```python
from build123d import *

# Parameters (mm, degrees)
ESTRUSIONE_ESTRUSIONE1_DEPTH = 60
SCHIZZO2_R                   = 2.6
TAGLIO_ESTRUSIONE1_DEPTH     = 60
SCHIZZO3_R                   = 2.4
TAGLIO_ESTRUSIONE2_DEPTH     = 10


with BuildPart() as part:
    # Schizzo1 → Estrusione-Estrusione1 (new body)
    with BuildSketch(Plane.XY):
        with BuildLine():
            Line((7.046874237, -2.567404038), (4.547114317, -1.124166975))
            Line((4.547114317, -1.124166975), (3.247114317, -3.375833025))
            Line((3.247114317, -3.375833025), (5.746874237, -4.819070087))
            ThreePointArc((5.746874237, -4.819070087), (0, -7.5), (-5.746874237, -4.819070087))
            Line((-5.746874237, -4.819070087), (-3.247114317, -3.375833025))
            Line((-3.247114317, -3.375833025), (-4.547114317, -1.124166975))
            Line((-4.547114317, -1.124166975), (-7.046874237, -2.567404038))
            ThreePointArc((-7.046874237, -2.567404038), (-6.495190528, 3.75), (-1.3, 7.386474125))
            Line((-1.3, 7.386474125), (-1.3, 4.5))
            Line((-1.3, 4.5), (1.3, 4.5))
            Line((1.3, 4.5), (1.3, 7.386474125))
            ThreePointArc((1.3, 7.386474125), (6.495190528, 3.75), (7.046874237, -2.567404038))
        make_face()
    extrude(amount=ESTRUSIONE_ESTRUSIONE1_DEPTH)

    # Schizzo2 → Taglio-Estrusione1 (cut)
    with BuildSketch(Plane.XY.offset(60)):
        Circle(SCHIZZO2_R)
    extrude(amount=-TAGLIO_ESTRUSIONE1_DEPTH, mode=Mode.SUBTRACT)

    # Schizzo3 → Taglio-Estrusione2 (cut)
    with BuildSketch(Plane(origin=(0, 0, 0), x_dir=(1, 0, 0), z_dir=(0, 1, 0))):
        with Locations(Location((0, -30, 0), (0, 0, 270))):
            Circle(SCHIZZO3_R)
    extrude(amount=-TAGLIO_ESTRUSIONE2_DEPTH, mode=Mode.SUBTRACT)


solid = part.part
```
Read the model definition and answer for the solid it produces. Units are mm, in the model's axes. A direction names the side the tool comes from. Round coordinates to 2 decimals unless told otherwise and drop trailing zeros. Write each loop counter-clockwise with the first axis right and the second up, starting at its lowest first coordinate (ties: lowest second). Pieces come first, ordered by that corner, then holes. Notation, with made-up numbers: (22.5, -16) - (80.5, -16) arc R18 ccw to (80.5, 5) - close; hole circle Ø3 at (-36, 0.25). An arc over 180 degrees is marked (long way). Use CSV: the item, a comma, the result in double quotes.
Q1. Each of these flat-tipped pins is pushed along its axis until it touches: pin 1 Ø1 at (x, z) = (-5.5, 10) entering from +Y; pin 2 Ø5 at (x, z) = (-4, 31) entering from -Y; pin 3 Ø0.9 at (y, z) = (6.5, 20) entering from -X; pin 4 Ø4 at (x, y) = (0, 0) entering from +Z. Where does it stop, or does it pass through?
Values:
pin 1,"stops at y = 5.59"
pin 2,"stops at y = -7.32"
pin 3,"stops at x = -4.43"
pin 4,"passes through"
Q2. Find section C-C, the plane z = 26. Write down the section's boundary in (x, y).
Values:
outline,"(-7.05, -2.57) - (-4.55, -1.12) - (-3.25, -3.38) - (-5.75, -4.82) arc R7.5 ccw to (5.75, -4.82) - (3.25, -3.38) - (4.55, -1.12) - (7.05, -2.57) arc R7.5 ccw to (1.3, 7.39) - (1.3, 4.5) - (-1.3, 4.5) - (-1.3, 7.39) arc R7.5 ccw to start; hole circle Ø5.2 at (0, 0)"
Q3. Find section B-B, the plane x = 0. Write down the section's boundary in (y, z), then the cut area to 3 significant figures.
Values:
outline,"(-7.5, 0) - (-2.6, 0) - (-2.6, 27.6) - (-7.5, 27.6) - close; (-7.5, 32.4) - (-2.6, 32.4) - (-2.6, 60) - (-7.5, 60) - close; (2.6, 0) - (4.5, 0) - (4.5, 60) - (2.6, 60) - close"
area,"384 mm²"
Q4. Find section A-A, the plane y = 0. Write down the section's boundary in (x, z), then the cut area to 3 significant figures.
Values:
outline,"(-7.5, 0) - (-2.6, 0) - (-2.6, 60) - (-7.5, 60) - close; (2.6, 0) - (7.5, 0) - (7.5, 60) - (2.6, 60) - close"
area,"588 mm²"
Q5. Straight lines are drawn through the part: line 1 along Z through (x, y) = (0, -4.5); line 2 along Y through (x, z) = (0, 26.5); line 3 along X through (y, z) = (-0.25, 54). For each, find the intervals that lie inside material, in ascending order.
Values:
line 1,"z = 0 to 27.6, 32.4 to 60"
line 2,"y = -7.5 to -2.6, 2.6 to 4.5"
line 3,"x = -7.5 to -2.59, 2.59 to 7.5"
Q6. A tool of negligible diameter and unlimited length cuts with its end or side. For faces 5 (the cylindrical face through (1.62, -4.93, 28.23)), 6 (the flat face through (1.3, 6, 30)), 7 (the flat face through (-4.5, -4.1, 29.6)), 8 (the flat face through (5.814, -1.856, 29.58)), from which of +Z, -Z, +X, -X, +Y, -Y can it reach the whole face along a straight path? Write none if from no direction.
Values:
face 5,"-Y"
face 6,"+Z, -Z, +Y"
face 7,"+Z, -Z, -X"
face 8,"+Z, -Z"
Q7. Determine the mould class of faces 1 (the flat face through (-3, 0, 0)), 2 (the cylindrical face through (-6.54, 3.67, 29.58)), 3 (the cylindrical face through (-2.752, -6.977, 29.58)), 4 (the flat face through (4.5, -4.1, 29.6)) for opening direction Y: +Y half, -Y half, draft (parallel to the pull), parting line (faces both ways), or undercut.
Values:
face 1,"draft"
face 2,"parting line"
face 3,"-Y half"
face 4,"undercut"
Q8. Find section D-D, the plane x = -4. Write down the section's boundary in (y, z).
Values:
outline,"(-6.34, 0) - (-3.81, 0) - (-3.81, 60) - (-6.34, 60) - close; (-2.07, 0) - (6.34, 0) - (6.34, 60) - (-2.07, 60) - close"
